Geometry: final body of the model. Coordinates: model frame, mm. A direction names the side the tool comes from. Give positions to 0.01 mm unless a question says otherwise; leave off trailing zeros. Loops run counter-clockwise (first coordinate to the right, second up) from the corner with the lowest first, then second, coordinate; pieces in that order, holes last. Notation, with made-up numbers: M 45.25,62.25 L 98.25,62.25 A13 cw 98.25,67.25 Z; hole C -31,46.5 d7. An arc over 180 degrees is marked long. Put each result on its own line as item: value.
Autodesk Inventor part; units mm, degrees
ref_plane "YZ Plane" through (0, 0, 0) normal (1, 0, 0) x (0, 1, 0)
ref_plane "XZ Plane" through (0, 0, 0) normal (0, 1, 0) x (-1, 0, 0)
ref_plane "XY Plane" through (0, 0, 0) normal (0, 0, 1) x (1, 0, 0)
sketch "Sketch1" plane through (0, 0, 0) normal (0, 0, 1) x (1, 0, 0)
  line L0 (-208.5912, 171.4818) -> (201.4088, 171.4818)
  line L1 (201.4088, 171.4818) -> (201.4088, -138.5182)
  line L2 (201.4088, -138.5182) -> (-208.5912, -138.5182)
  line L3 (-208.5912, -138.5182) -> (-208.5912, 171.4818)
  line L4 (-248.5912, 201.4818) -> (241.4088, 201.4818)
  line L5 (241.4088, 201.4818) -> (241.4088, -188.5182)
  line L6 (241.4088, -188.5182) -> (-248.5912, -188.5182)
  line L7 (-248.5912, -188.5182) -> (-248.5912, 201.4818)
  point P0 (0, 0)
  dimension "d0" = 410
  dimension "d1" = 310
  dimension "d2" = 490
  dimension "d3" = 40
  dimension "d4" = 390
  dimension "d5" = 50
extrude "Extrusion1" add sketch "Sketch1" along normal blind 15
sketch "Sketch2" plane through (241.4088, -188.5182, 0) normal (1, 0, 0) x (0, 0, -1)
  line L0 (0, 390) -> (-15, 390)
  line L1 (0, 390) -> (-5, 390)
  line L2 (-5, 390) -> (-5, 0)
  line L3 (-5, 0) -> (0, 0)
  line L4 (0, 0) -> (0, 390)
  point P0 (0, 188.5182)
  dimension "d8" = 5
  dimension "d9" = 390
extrude "Extrusion2" cut sketch "Sketch2" against normal blind 7
sketch "Sketch3" plane through (-248.5912, -188.5182, 0) normal (-1, 0, 0) x (0, 0, 1)
  line L0 (0, 390) -> (0, 0)
  line L1 (5, 0) -> (5, 390)
  line L2 (0, 390) -> (5, 390)
  line L3 (5, 390) -> (5, 0)
  line L4 (5, 0) -> (0, 0)
  line L5 (0, 0) -> (0, 390)
  point P0 (0, 188.5182)
  point P1 (0, 0)
  dimension "d12" = 5
  dimension "d13" = 390
extrude "Extrusion3" cut sketch "Sketch3" against normal blind 7
sketch "Sketch4" plane through (0, 0, 0) normal (0, 0, -1) x (-1, 0, 0)
  line L0 (-234.4088, 201.4818) -> (241.5912, 201.4818)
  line L1 (-234.4088, 201.4818) -> (241.5912, 201.4818)
  line L2 (241.5912, 201.4818) -> (241.5912, -188.5182)
  line L3 (241.5912, -188.5182) -> (-234.4088, -188.5182)
  line L4 (-234.4088, -188.5182) -> (-234.4088, 201.4818)
  line L5 (208.5912, 171.4818) -> (-201.4088, 171.4818)
  line L6 (-201.4088, 171.4818) -> (208.5912, 171.4818)
  line L7 (208.5912, 171.4818) -> (208.5912, -138.5182)
  line L8 (208.5912, -138.5182) -> (-201.4088, -138.5182)
  line L9 (-201.4088, -138.5182) -> (-201.4088, 171.4818)
  point P0 (0, 0)
extrude "Extrusion4" add sketch "Sketch4" along normal blind 1
properties part number "Arcade_Front"
Item 1: Section B-B on x = -10. Output: boundary loops of the cut face in (y, z).
Output values:
outline: M -188.52,-1 L -138.52,-1 L -138.52,15 L -188.52,15 Z; M 171.48,-1 L 201.48,-1 L 201.48,15 L 171.48,15 Z
Item 2: Line query: probe 1 along Y at (x, z) = (-63, 11.25); probe 2 along X at (y, z) = (-100, 10.5); probe 3 along X at (y, z) = (-107, 2.25). Output: solid intervals per line, ascending. Write a range as [from, to].
Output values:
probe 1: [-188.52, -138.52], [171.48, 201.48]
probe 2: [-248.59, -208.59], [201.41, 241.41]
probe 3: [-241.59, -208.59], [201.41, 234.41]
Item 3: Section C-C on z = 10.75. Output: boundary loops of the cut face in (x, y).
Output values:
outline: M -248.59,-188.52 L 241.41,-188.52 L 241.41,201.48 L -248.59,201.48 Z; hole M -208.59,-138.52 L 201.41,-138.52 L 201.41,171.48 L -208.59,171.48 Z
Item 4: Mould query, pull axis X, two halves, no side actions, for faces 1 (the flat face through (0, 201.482, 7)), 2 (the flat face through (-248.591, 4, 10)), 3 (the flat face through (-208.591, 19, 7)), 4 (the flat face through (241.409, 9, 10)). Classes: pulls with the +X half, pulls with the -X half, needs draft (parallel to the pull), parting line crosses it, or undercut.
Output values:
face 1: needs draft
face 2: pulls with the -X half
face 3: undercut
face 4: pulls with the +X half
Item 5: Section A-A on y = 65. Output: boundary loops of the cut face in (x, z).
Output values:
outline: M -248.59,5 L -241.59,5 L -241.59,-1 L -208.59,-1 L -208.59,15 L -248.59,15 Z; M 201.41,-1 L 234.41,-1 L 234.41,5 L 241.41,5 L 241.41,15 L 201.41,15 Z
Item 6: Set-up query: faces 5 (the flat face through (-7, -188.518, 7)), 6 (the flat face through (-6, 171.482, 7)). Return all of +Z, -Z, +X, -X, +Y, -Y with unobstructed straight access to the full face (end or side cutting, diameter ignored); none if empty.
Output values:
face 5: +Z, -Z, +X, -X, -Y
face 6: +Z, -Z
Item 7: Pin query (flat end, axial travel): pin 1 Ø1.8 at (y, z) = (-12, 2) entering from +X; pin 2 Ø3.5 at (x, y) = (239, -49) entering from -Z; pin 3 Ø6 at (y, z) = (65, 1) entering from -X. Return the tip coordinate at first contact, or that it passes through.
Output values:
pin 1: x = 234.41
pin 2: z = 5
pin 3: x = -241.59
